```python
from build123d import *

# Parameters (mm, degrees)
F0_W         = 127
F0_H         = 76.2
F0_R         = 6.35
F1_DEPTH     = 12.7
F2_R         = 5.08
F3_T1_DEPTH  = 20.32
F3_S5_W      = 5.08
F3_S5_H      = 5.08
F3_T6_DEPTH  = 5.08
F3_S11_W     = 5.08
F3_S11_H     = 5.08
F3_T12_DEPTH = 5.08
F3_S17_W     = 5.08
F3_S17_H     = 5.08
F3_T18_DEPTH = 5.08
F3_S23_W     = 5.08
F3_S23_H     = 5.08
F3_T24_DEPTH = 5.08
F4_W         = 5.08
F4_H         = 5.08
F5_DEPTH     = 76.2


# Not quite as in the source:
# - a fillet or chamfer that OpenCascade refuses, or shapes differently, is made with other operations: its cross-section is extruded or revolved along the edge and cut away or added


with BuildPart() as f1:
    # F0 (on Front) → F1 (new body)
    with BuildSketch(Plane.XZ):
        with Locations((-0.4540607333, -4.4948741291)):
            Rectangle(F0_W, F0_H)
        with Locations((-38.5540607333, -23.5448741291)):
            Circle(F0_R, mode=Mode.SUBTRACT)
        with Locations((-0.4540607333, -23.5448741291)):
            Circle(F0_R, mode=Mode.SUBTRACT)
        with Locations((37.6459392667, -23.5448741291)):
            Circle(F0_R, mode=Mode.SUBTRACT)
        with Locations((-38.5540607333, 14.5551258709)):
            Circle(F0_R, mode=Mode.SUBTRACT)
        with Locations((-0.4540607333, 14.5551258709)):
            Circle(F0_R, mode=Mode.SUBTRACT)
        with Locations((37.6459392667, 14.5551258709)):
            Circle(F0_R, mode=Mode.SUBTRACT)
    extrude(amount=F1_DEPTH)

    # F2
    f2_edges = [f1.edges().sort_by_distance(p)[0] for p in [
        (-0.454061, -12.7, 33.605126),
        (-63.954061, -12.7, -4.494874),
        (-0.454061, -12.7, -42.594874),
        (63.045939, -12.7, -4.494874),
    ]]
    fillet(f2_edges, radius=F2_R)

    # F3: fillet of radius 5.08 on 4 edges, made by hand

    # F3_s2 → F3_t1 (cut)
    with BuildSketch(Plane.XZ.offset(-12.7)):
        with BuildLine():
            ThreePointArc((-63.9540607333, -37.5148741291), (-62.4661631817, -41.1069765775), (-58.8740607333, -42.5948741291))
            Line((-58.8740607333, -42.5948741291), (-63.9540607333, -42.5948741291))
            Line((-63.9540607333, -42.5948741291), (-63.9540607333, -37.5148741291))
        make_face()
        with BuildLine():
            ThreePointArc((63.0459392667, -37.5148741291), (61.5580417151, -41.1069765775), (57.9659392667, -42.5948741291))
            Line((57.9659392667, -42.5948741291), (63.0459392667, -42.5948741291))
            Line((63.0459392667, -42.5948741291), (63.0459392667, -37.5148741291))
        make_face()
        with BuildLine():
            ThreePointArc((57.9659392667, 33.6051258709), (61.5580417151, 32.1172283193), (63.0459392667, 28.5251258709))
            Line((63.0459392667, 28.5251258709), (63.0459392667, 33.6051258709))
            Line((63.0459392667, 33.6051258709), (57.9659392667, 33.6051258709))
        make_face()
        with BuildLine():
            ThreePointArc((-58.8740607333, 33.6051258709), (-62.4661631817, 32.1172283193), (-63.9540607333, 28.5251258709))
            Line((-63.9540607333, 28.5251258709), (-63.9540607333, 33.6051258709))
            Line((-63.9540607333, 33.6051258709), (-58.8740607333, 33.6051258709))
        make_face()
    extrude(amount=F3_T1_DEPTH, mode=Mode.SUBTRACT)


with BuildPart() as f3_tool4:
    # F3_s5 → F3_t6 (new body)
    with BuildSketch(Plane.XY.offset(28.5251258709)):
        with Locations((-61.4140607333, -10.16)):
            Rectangle(F3_S5_W, F3_S5_H)
    extrude(amount=F3_T6_DEPTH)

    # F3_s7 → F3_t8 (revolve, cut)
    with BuildSketch(Plane(origin=(-58.8740607333, -7.62, 28.5251258709), x_dir=(0.7071067812, 0.7071067812, 0), z_dir=(0.7071067812, -0.7071067812, 0))):
        with BuildLine():
            ThreePointArc((0, -5.08), (5.08, 0), (0, 5.08))
            Line((0, 5.08), (0, -5.08))
        make_face()
    revolve(axis=Axis((-58.8740607333, -7.62, 28.5251258709), (0, 0, 1)), mode=Mode.SUBTRACT)


with BuildPart() as f1_1:
    add(f1.part)

    # F3_t3: cut F3_tool4
    add(f3_tool4.part, mode=Mode.SUBTRACT)


with BuildPart() as f3_tool10:
    # F3_s11 → F3_t12 (new body)
    with BuildSketch(Plane.XY.offset(28.5251258709)):
        with Locations((60.5059392667, -10.16)):
            Rectangle(F3_S11_W, F3_S11_H)
    extrude(amount=F3_T12_DEPTH)

    # F3_s13 → F3_t14 (revolve, cut)
    with BuildSketch(Plane(origin=(57.9659392667, -7.62, 28.5251258709), x_dir=(-0.7071067812, 0.7071067812, 0), z_dir=(0.7071067812, 0.7071067812, 0))):
        with BuildLine():
            ThreePointArc((0, -5.08), (5.08, 0), (0, 5.08))
            Line((0, 5.08), (0, -5.08))
        make_face()
    revolve(axis=Axis((57.9659392667, -7.62, 28.5251258709), (0, 0, 1)), mode=Mode.SUBTRACT)


with BuildPart() as f1_2:
    add(f1_1.part)

    # F3_t9: cut F3_tool10
    add(f3_tool10.part, mode=Mode.SUBTRACT)


with BuildPart() as f3_tool16:
    # F3_s17 → F3_t18 (new body)
    with BuildSketch(Plane.YZ.offset(57.9659392667)):
        with Locations((-10.16, -40.0548741291)):
            Rectangle(F3_S17_W, F3_S17_H)
    extrude(amount=F3_T18_DEPTH)

    # F3_s19 → F3_t20 (revolve, cut)
    with BuildSketch(Plane(origin=(57.9659392667, -7.62, -37.5148741291), x_dir=(0, 0.7071067812, 0.7071067812), z_dir=(0, 0.7071067812, -0.7071067812))):
        with BuildLine():
            ThreePointArc((0, -5.08), (5.08, 0), (0, 5.08))
            Line((0, 5.08), (0, -5.08))
        make_face()
    revolve(axis=Axis((57.9659392667, -7.62, -37.5148741291), (1, 0, 0)), mode=Mode.SUBTRACT)


with BuildPart() as f1_3:
    add(f1_2.part)

    # F3_t15: cut F3_tool16
    add(f3_tool16.part, mode=Mode.SUBTRACT)


with BuildPart() as f3_tool22:
    # F3_s23 → F3_t24 (new body)
    with BuildSketch(Plane.YZ.offset(-58.8740607333)):
        with Locations((-10.16, -40.0548741291)):
            Rectangle(F3_S23_W, F3_S23_H)
    extrude(amount=-F3_T24_DEPTH)

    # F3_s25 → F3_t26 (revolve, cut)
    with BuildSketch(Plane(origin=(-58.8740607333, -7.62, -37.5148741291), x_dir=(0, 0.7071067812, 0.7071067812), z_dir=(0, -0.7071067812, 0.7071067812))):
        with BuildLine():
            ThreePointArc((0, -5.08), (5.08, 0), (0, 5.08))
            Line((0, 5.08), (0, -5.08))
        make_face()
    revolve(axis=Axis((-58.8740607333, -7.62, -37.5148741291), (-1, 0, 0)), mode=Mode.SUBTRACT)


with BuildPart() as f1_4:
    add(f1_3.part)

    # F3_t21: cut F3_tool22
    add(f3_tool22.part, mode=Mode.SUBTRACT)

    # F4 (on face) → F5 (join)
    with BuildSketch(Plane.XZ.offset(12.7)):
        with Locations((-56.3340607333, -34.9748741291)):
            Rectangle(F4_W, F4_H)
        with Locations((55.4259392667, -34.9748741291)):
            Rectangle(F4_W, F4_H)
        with Locations((55.4259392667, 25.9851258709)):
            Rectangle(F4_W, F4_H)
        with Locations((-56.3340607333, 25.9851258709)):
            Rectangle(F4_W, F4_H)
    extrude(amount=F5_DEPTH)


solid = f1_4.part
```
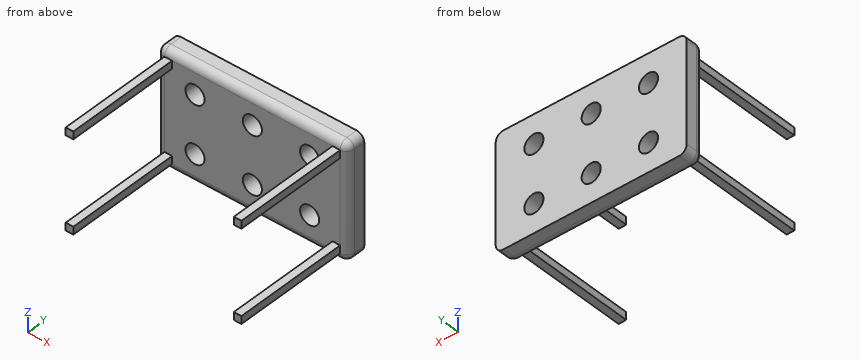
Build history of the part. All positions in model axes, mm. Give positions to 0.01 mm unless a question says otherwise; leave off trailing zeros. Loops run counter-clockwise (first coordinate to the right, second up) from the corner with the lowest first, then second, coordinate; pieces in that order, holes last.
1) Band-saw the part on D-D on x = 18. List the corners of the cut face in (y, z).
Values follow:
outline: (-12.7, -37.51) arc R5.08 ccw to (-7.62, -42.59) - (0, -42.59) - (0, 33.61) - (-7.62, 33.61) arc R5.08 ccw to (-12.7, 28.53) - close
2) Band-saw the part on B-B on z = -20. List the corners of the cut face in (x, y).
Values follow:
outline: (-63.95, -7.62) arc R5.08 ccw to (-58.87, -12.7) - (-43.82, -12.7) - (-43.82, 0) - (-63.95, 0) - close; (-33.29, -12.7) - (-5.72, -12.7) - (-5.72, 0) - (-33.29, 0) - close; (4.81, -12.7) - (32.38, -12.7) - (32.38, 0) - (4.81, 0) - close; (42.91, -12.7) - (57.97, -12.7) arc R5.08 ccw to (63.05, -7.62) - (63.05, 0) - (42.91, 0) - close
3) Drop flat-ended pins along their axis: P1, Ø10, axis at x = 0, z = -20, coming from the -Y side; P2, Ø4, axis at x = -57.5, y = -59, coming from the +Z side; P3, Ø2.5, axis at x = 55.5, y = -54, coming from the -Z side. Give the stop position or say it passes through.
Values follow:
P1: stops at y = -12.7
P2: stops at z = 28.53
P3: stops at z = -37.51
4) Band-saw the part on C-C on x = -36.5. List the corners of the cut face in (y, z), then the cut area to 3 significant figures.
Values follow:
outline: (-12.7, -37.51) arc R5.08 ccw to (-7.62, -42.59) - (0, -42.59) - (0, -29.55) - (-12.7, -29.55) - close; (-12.7, -17.54) - (0, -17.54) - (0, 8.55) - (-12.7, 8.55) - close; (-12.7, 20.56) - (0, 20.56) - (0, 33.61) - (-7.62, 33.61) arc R5.08 ccw to (-12.7, 28.53) - close
area: 651 mm2
5) Band-saw the part on A-A on y = -67.5. List the corners of the cut face in (x, z), then the cut area to 3 significant figures.
Values follow:
outline: (-58.87, -37.51) - (-53.79, -37.51) - (-53.79, -32.43) - (-58.87, -32.43) - close; (-58.87, 23.45) - (-53.79, 23.45) - (-53.79, 28.53) - (-58.87, 28.53) - close; (52.89, -37.51) - (57.97, -37.51) - (57.97, -32.43) - (52.89, -32.43) - close; (52.89, 23.45) - (57.97, 23.45) - (57.97, 28.53) - (52.89, 28.53) - close
area: 103 mm2
6) Probe line 1 along X through (y, z) = (-52.5, -33.5); line 2 along Y through (x, z) = (-29.5, 27.5); line 3 along Z through (x, y) = (0.5, -7.5). List the from-to ranges inside material, lowest first.
Values follow:
line 1: x = -58.87 to -53.79, 52.89 to 57.97
line 2: y = -12.7 to 0
line 3: z = -42.59 to -29.82, -17.27 to 8.28, 20.83 to 33.61
